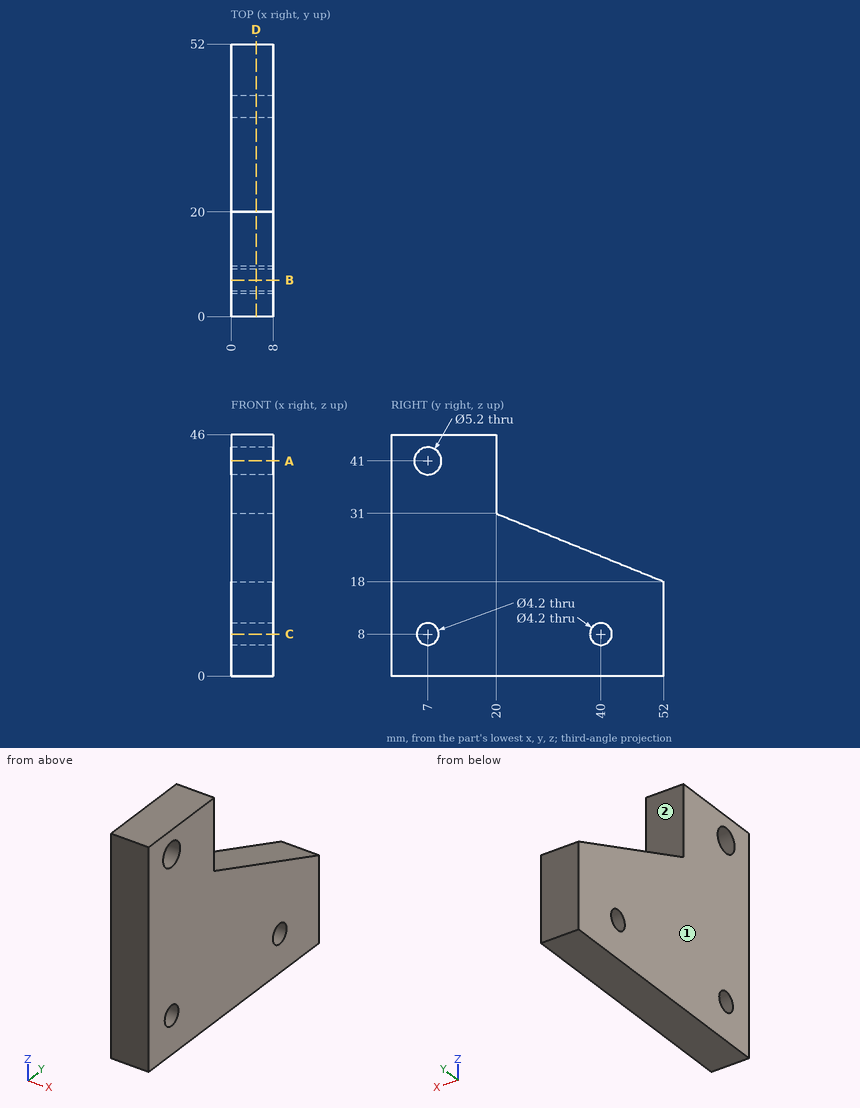
Geometry check sheet. Reference: drawing and pictorial views, mm from the part's lowest x, y, z. A direction names the side the tool comes from. Give positions to 0.01 mm unless a question says otherwise; leave off trailing zeros. Loops run counter-clockwise (first coordinate to the right, second up) from the corner with the lowest first, then second, coordinate; pieces in that order, holes last. Notation, with made-up numbers: (84.25, 85) -> (93.25, 85) arc R29 cw to (93.25, 110) -> close; hole circle Ø9 at (85.25, 61). An arc over 180 degrees is marked (long way). Answer in a Markdown table with one row per item. Add a question column.
1) Material ranges on probe 1 along Z at (x, y) = (3.75, 7); probe 2 along Y at (x, z) = (4, 32); probe 3 along Y at (x, z) = (2.75, 9), recorded low to high. Write a range as from..to.
2) Cross-section at D-D on x = 4.75. Record the boundary of the cut face in (y, z), and give its area (3 significant figures).
3) Set-up check for the marked faces 1 and 2: record each of +Z, -Z, +X, -X, +Y, -Y from which the full face is reachable in a straight line by a thin tool's end or side.
4) Gauge pin test, flat ends, axial feed: P1, Ø2, axis at y = 17, z = 26, coming from the -X side; P2, Ø2.5, axis at x = 3, z = 35, coming from the +Y side. Record the tip position at first contact, or that the pin passes through.
5) Cross-section at A-A on z = 41. Record the boundary of the cut face in (x, y), and give its area (3 significant figures).
6) Cross-section at B-B on y = 7. Record the boundary of the cut face in (x, z), and give its area (3 significant figures).
7) Cross-section at C-C on z = 8. Record the boundary of the cut face in (x, y).
Outcome:
| question | item | result |
|---|---|---|
| 1 | probe 1 | z = 0..5.9, 10.1..38.4, 43.6..46 |
| 1 | probe 2 | y = 0..20 |
| 1 | probe 3 | y = 0..5.15, 8.85..38.15, 41.85..52 |
| 2 | outline | (0, 0) -> (52, 0) -> (52, 18) -> (20, 31) -> (20, 46) -> (0, 46) -> close; hole circle Ø5.2 at (7, 41); hole circle Ø4.2 at (7, 8); hole circle Ø4.2 at (40, 8) |
| 2 | area | 1,660 mm^2 |
| 3 | face 1 | +Z, -Z, -X, +Y, -Y |
| 3 | face 2 | +Z, +X, -X, +Y |
| 4 | P1 | stops at x = 0 |
| 4 | P2 | stops at y = 20 |
| 5 | outline | (0, 0) -> (8, 0) -> (8, 4.4) -> (0, 4.4) -> close; (0, 9.6) -> (8, 9.6) -> (8, 20) -> (0, 20) -> close |
| 5 | area | 118 mm^2 |
| 6 | outline | (0, 0) -> (8, 0) -> (8, 5.9) -> (0, 5.9) -> close; (0, 10.1) -> (8, 10.1) -> (8, 38.4) -> (0, 38.4) -> close; (0, 43.6) -> (8, 43.6) -> (8, 46) -> (0, 46) -> close |
| 6 | area | 293 mm^2 |
| 7 | outline | (0, 0) -> (8, 0) -> (8, 4.9) -> (0, 4.9) -> close; (0, 9.1) -> (8, 9.1) -> (8, 37.9) -> (0, 37.9) -> close; (0, 42.1) -> (8, 42.1) -> (8, 52) -> (0, 52) -> close |
